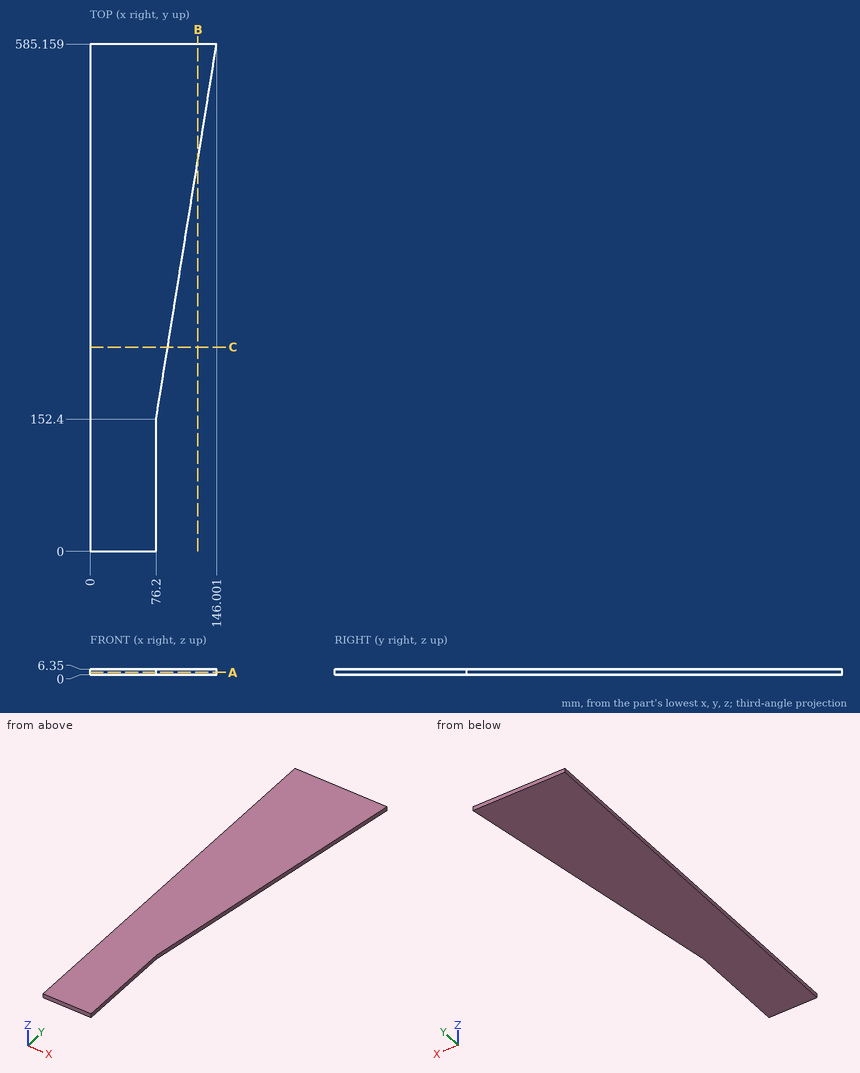
Geometry check sheet. Reference: drawing and pictorial views, mm from the part's lowest x, y, z. Round coordinates to 2 decimals unless told otherwise and drop trailing zeros. Loops run counter-clockwise (first coordinate to the right, second up) from the corner with the lowest first, then second, coordinate; pieces in that order, holes last. Notation, with made-up numbers: (34.5, 28) -> (61.5, 28) arc R11 cw to (61.5, 41) -> close; hole circle Ø3 at (-20, 2). An arc over 180 degrees is marked (long way). Answer as a JSON object with one key per item and string values. Group by question number.
Item 1: Thickness scan on line 1 along X through (y, z) = (63.5, 6.25); line 2 along X through (y, z) = (545, 2). Record the ranges inside material, lowest first.
Item 2: Cross-section at B-B, the plane x = 124.5. Record the cut outline in (y, z).
Item 3: Depth check by flat-ended pin: pin 1 Ø3 at (y, z) = (210, 3) entering from -X; pin 2 Ø3 at (y, z) = (328.5, 2.5) entering from +X. Enter the tip coordinate at first touch or a pass-through.
Item 4: Cross-section at A-A, the plane z = 3. Record the cut outline in (x, y).
Item 5: Cross-section at C-C, the plane y = 235.5. Record the cut outline in (x, z), plus the area to 3 significant figures.
Determined:
{
 "1": {"line 1": "x = 0 to 76.2", "line 2": "x = 0 to 139.52"},
 "2": {"outline": "(451.85, 0) -> (585.16, 0) -> (585.16, 6.35) -> (451.85, 6.35) -> close"},
 "3": {"pin 1": "stops at x = 0", "pin 2": "stops at x = 104.85"},
 "4": {"outline": "(0, 0) -> (76.2, 0) -> (76.2, 152.4) -> (146, 585.16) -> (0, 585.16) -> close"},
 "5": {"outline": "(0, 0) -> (89.6, 0) -> (89.6, 6.35) -> (0, 6.35) -> close", "area": "569 mm²"}
}
